from build123d import *

# Parameters (mm, degrees)
SKETCH1_W               = 127
SKETCH1_H               = 127
BOSS_EXTRUDE1_DEPTH     = 76.2
SHELL2_T                = -2.54
CUT_EXTRUDE1_DEPTH      = 162.144934764
CUT_EXTRUDE1_DEPTH_BACK = 2.54
FILLET3_R               = 2.54
SKETCH3_R               = 1.4097
CUT_EXTRUDE2_DEPTH      = 162.144934764


with BuildPart() as part:
    # Sketch1 → Boss-Extrude1 (new body)
    with BuildSketch(Plane.XY):
        Rectangle(SKETCH1_W, SKETCH1_H)
    extrude(amount=BOSS_EXTRUDE1_DEPTH)

    # Shell2
    shell2_openings = [part.faces().sort_by_distance(p)[0] for p in [
        (0, 0, 0),
    ]]
    offset(amount=SHELL2_T, openings=shell2_openings, kind=Kind.INTERSECTION)

    # Sketch2 → Cut-Extrude1 (cut, two sides: drawn at the far end of the back side and taken through both)
    with BuildSketch(Plane(origin=(0, 63.5, 0), x_dir=(1, 0, 0), z_dir=(0, 1, 0)).offset(-CUT_EXTRUDE1_DEPTH_BACK)):
        with BuildLine():
            Line((-12.7, 225.526146906), (-12.7, 0))
            ThreePointArc((-12.7, 0), (0, -12.7), (12.7, 0))
            Line((12.7, 0), (12.7, 225.526146906))
            Line((12.7, 225.526146906), (12.7, 676.578440717))
            Line((12.7, 676.578440717), (-12.7, 676.578440717))
            Line((-12.7, 676.578440717), (-12.7, 225.526146906))
        make_face()
    extrude(amount=CUT_EXTRUDE1_DEPTH + CUT_EXTRUDE1_DEPTH_BACK, mode=Mode.SUBTRACT)

    # Fillet3
    # the kernel refuses this fillet: 2.54 mm, written as the material it takes off along each edge
    with BuildSketch(Plane(origin=(0, 60.96, 0), x_dir=(-0.8771967747646356, 0, -0.4801310428857115), z_dir=(0.4801310428857115, 0, -0.8771967747646356))) as fillet3_piece_1:
        with BuildLine():
            CenterArc((12.7 + FILLET3_R, FILLET3_R), FILLET3_R, 180, 90)
            Line((12.7 + FILLET3_R, 0), (12.7, 0))
            Line((12.7, 0), (12.7, FILLET3_R))
        make_face()
    revolve(axis=Axis((0, 60.96, 0), (0, 1, 0)), revolution_arc=237.38792196, mode=Mode.SUBTRACT)
    with BuildSketch(Plane(origin=(0, 63.5, 0), x_dir=(0.8771967747646356, 0, -0.4801310428857116), z_dir=(-0.4801310428857116, 0, -0.8771967747646356))) as fillet3_piece_2:
        with BuildLine():
            CenterArc((12.7 + FILLET3_R, FILLET3_R), FILLET3_R, 180, 90)
            Line((12.7, FILLET3_R), (12.7, 0))
            Line((12.7, 0), (12.7 + FILLET3_R, 0))
        make_face()
    revolve(axis=Axis((0, 63.5, 0), (0, -1, 0)), revolution_arc=237.38792196, mode=Mode.SUBTRACT)

    # Sketch3 → Cut-Extrude2 (cut, through all)
    with BuildSketch(Plane.XZ.offset(63.5)):
        with Locations(Location((-55.88, 20.32, 0), (0, 0, 270))):
            Circle(SKETCH3_R)
        with Locations(Location((-45.72, 20.32, 0), (0, 0, 270))):
            Circle(SKETCH3_R)
        with Locations(Location((-55.88, 10.16, 0), (0, 0, 270))):
            Circle(SKETCH3_R)
        with Locations(Location((-45.72, 10.16, 0), (0, 0, 270))):
            Circle(SKETCH3_R)
    cut_extrude2 = extrude(amount=-CUT_EXTRUDE2_DEPTH, mode=Mode.SUBTRACT)

    # Mirror1: Cut-Extrude2 across plane
    add(cut_extrude2.mirror(Plane(origin=(0, 0, 0), x_dir=(0, 0, 1), z_dir=(1, 0, 0))), mode=Mode.SUBTRACT)


solid = part.part
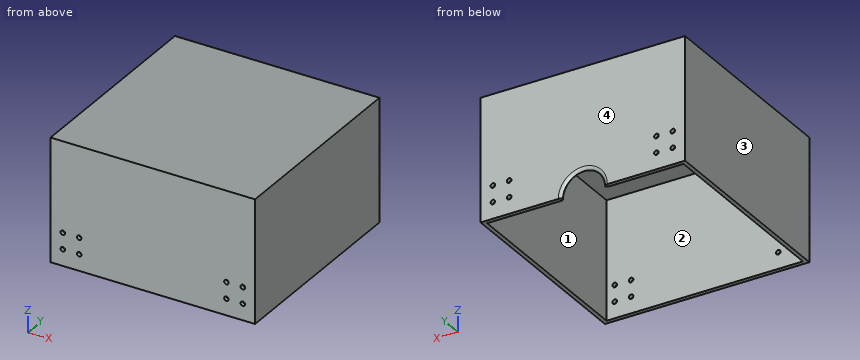
Check sheet for the modelled part. Datum: model origin and axes. Units: mm. Face numbers are marked on the shaded views. Round coordinates to 2 decimals unless told otherwise and drop trailing zeros. Loops run counter-clockwise (first coordinate to the right, second up) from the corner with the lowest first, then second, coordinate; pieces in that order, holes last.
1. Mould release check, pull along X, two halves, no side actions. Record for the marked faces 1, 2, 3 and 4: released by +X, released by -X, zero draft, split by the parting line, or undercut.
2. Scan lines: probe 1 along X at (y, z) = (62.3, 20.32); probe 2 along Z at (x, y) = (45.72, -62.45); probe 3 along X at (y, z) = (-58, 42). Record each from-to range of solid material in increasing order.
3. Gauge pin test, flat ends, axial feed: pin 1 Ø1.7 at (x, z) = (55.88, 10.16) entering from -Y; pin 2 Ø3 at (x, z) = (-45.72, 20.32) entering from +Y. Record the tip position at first contact, or that the pin passes through.
4. Sectioned sample at A-A on z = 70.5. Record the boundary of the cut face in (x, y), and give its area (3 significant figures).
5. Sectioned sample at B-B on x = 29.5. Record the boundary of the cut face in (y, z), and give its area (3 significant figures).
Recorded:
1. face 1: undercut
1. face 2: undercut
1. face 3: released by -X
1. face 4: zero draft
2. probe 1: x = -63.5 to -57.29, -54.47 to -47.13, -44.31 to 44.31, 47.13 to 54.47, 57.29 to 63.5
2. probe 2: z = 0 to 8.75, 11.57 to 18.91, 21.73 to 76.2
2. probe 3: x = -63.5 to -60.96, 60.96 to 63.5
3. pin 1: passes through
3. pin 2: stops at y = 63.5
4. outline: (-63.5, -63.5) - (63.5, -63.5) - (63.5, 63.5) - (-63.5, 63.5) - close; hole (-60.96, -60.96) - (60.96, -60.96) - (60.96, 60.96) - (-60.96, 60.96) - close
4. area: 1,260 mm2
5. outline: (-63.5, 0) - (-60.96, 0) - (-60.96, 73.66) - (60.96, 73.66) - (60.96, 0) - (63.5, 0) - (63.5, 76.2) - (-63.5, 76.2) - close
5. area: 697 mm2
